Could you check a few things on this model? Use its own coordinates, in mm. Give positions to 0.01 mm unless a question says otherwise; leave off trailing zeros. Loops run counter-clockwise (first coordinate to the right, second up) from the corner with the lowest first, then second, coordinate; pieces in that order, holes last. Notation, with made-up numbers: M -26,58.5 L 29,58.5 A21 ccw 29,70.5 Z; hole C 22.5,48 d6. An arc over 180 degrees is marked long. Use a Markdown table: item, result. Add a question column.
1) Suppose I cut it at D-D on z = -38. List the corners of the cut face in (x, y) for me.
2) Will these pins go through, and if not, where does the flat tip stop? pin 1 Ø3 at (x, z) = (-26, -39.5) entering from +Y; pin 2 Ø2 at (y, z) = (-1.5, 27.5) entering from -X; pin 3 Ø3 at (y, z) = (-2, -8.5) entering from -X; pin 4 Ø6 at (x, z) = (40.58, 46.87) entering from +Y.
3) Suppose I cut it at A-A on x = 0. List the corners of the cut face in (y, z) for me.
4) If I drill on line 1 along Z through (x, y) = (0, -4.3); line 2 along Z through (x, y) = (0, -2.75); line 3 along Z through (x, y) = (-42.5, -3.3), over which ranges is the centre line in solid material (lowest first)? Write a range as [from, to].
5) Suppose I cut it at C-C on y = -0.8. List the corners of the cut face in (x, z) for me, and give its area (3 significant figures).
6) Suppose I cut it at B-B on z = 0. List the corners of the cut face in (x, y) for me.
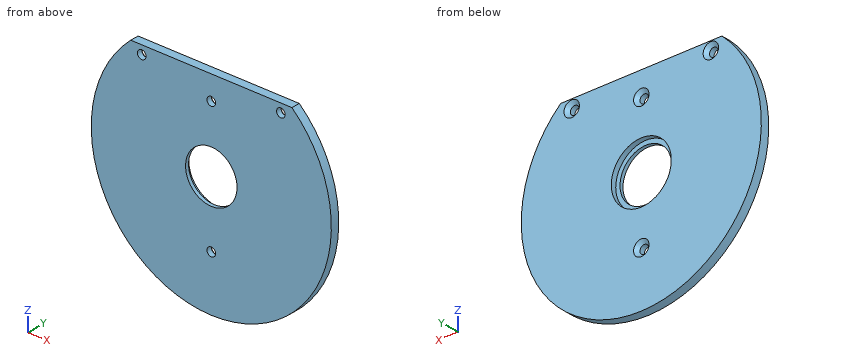
```python
from build123d import *

# Parameters (mm, degrees)
F2_R           = 2.5
F2_R_2         = 17.5
F2_R_3         = 15
F3_DEPTH       = 5
F4_DEPTH       = 3
F5_D           = 5
F5_CSINK_D     = 9
F5_CSINK_ANGLE = 90


with BuildPart() as f3:
    # F2 (on Front) → F3 (new body)
    with BuildSketch(Plane.XZ):
        with BuildLine():
            Line((47, 51.8748493974), (-47, 51.8748493974))
            ThreePointArc((-47, 51.8748493974), (0, -70), (47, 51.8748493974))
        make_face()
        with Locations((0, -38)):
            Circle(F2_R, mode=Mode.SUBTRACT)
        with Locations((-40.5801490137, 46.8748493974)):
            Circle(F2_R, mode=Mode.SUBTRACT)
        Circle(F2_R_2, mode=Mode.SUBTRACT)
        with Locations((0, 38)):
            Circle(F2_R, mode=Mode.SUBTRACT)
        with Locations((40.5801490137, 46.8748493974)):
            Circle(F2_R, mode=Mode.SUBTRACT)
        with Locations((40.5801490137, 46.8748493974)):
            Circle(F2_R)
        with Locations((0, 38)):
            Circle(F2_R)
        with Locations((-40.5801490137, 46.8748493974)):
            Circle(F2_R)
        with Locations((0, -38)):
            Circle(F2_R)
        Circle(F2_R_2)
        Circle(F2_R_3, mode=Mode.SUBTRACT)
    extrude(amount=F3_DEPTH)

    # F2 (on Front) → F4 (cut)
    with BuildSketch(Plane.XZ):
        Circle(F2_R_2)
        Circle(F2_R_3, mode=Mode.SUBTRACT)
    extrude(amount=F4_DEPTH, mode=Mode.SUBTRACT)

    # F5 (through all)
    with Locations(Plane(origin=(0, 0, 0), x_dir=(1, 0, 0), z_dir=(0, 1, 0))):
        with Locations((-40.5801490137, -46.8748493974), (0, -38), (40.5801490137, -46.8748493974), (0, 38)):
            CounterSinkHole(F5_D / 2, F5_CSINK_D / 2, counter_sink_angle=F5_CSINK_ANGLE)


solid = f3.part
```
Answer block:
| question | item | result |
|---|---|---|
| 1 | outline | M -58.79,-5 L -2.5,-5 L -2.5,-2 L -4.5,0 L -58.79,0 Z; M 2.5,-5 L 58.79,-5 L 58.79,0 L 4.5,0 L 2.5,-2 Z |
| 2 | pin 1 | stops at y = 0 |
| 2 | pin 2 | stops at x = -64.79 |
| 2 | pin 3 | stops at x = -69.65 |
| 2 | pin 4 | stops at y = -1.5 |
| 3 | outline | M -5,-70 L 0,-70 L 0,-42.5 L -2,-40.5 L -5,-40.5 Z; M -5,-35.5 L -2,-35.5 L 0,-33.5 L 0,-17.5 L -3,-17.5 L -3,-15 L -5,-15 Z; M -5,15 L -3,15 L -3,17.5 L 0,17.5 L 0,33.5 L -2,35.5 L -5,35.5 Z; M -5,40.5 L -2,40.5 L 0,42.5 L 0,51.87 L -5,51.87 Z |
| 4 | line 1 | z = [-70, -40.5], [-35.5, -15], [15, 35.5], [40.5, 51.87] |
| 4 | line 2 | z = [-70, -40.5], [-35.5, -17.5], [17.5, 35.5], [40.5, 51.87] |
| 4 | line 3 | z = [-55.62, 45.27], [48.48, 51.87] |
| 5 | outline | M -47,51.87 A70 ccw long 47,51.87 Z; hole C -40.58,46.87 d7.4; hole C 0,0 d35; hole C 0,-38 d7.4; hole C 0,38 d7.4; hole C 40.58,46.87 d7.4 |
| 5 | area | 13,100 mm^2 |
| 6 | outline | M -70,-5 L -15,-5 L -15,-3 L -17.5,-3 L -17.5,0 L -70,0 Z; M 15,-5 L 70,-5 L 70,0 L 17.5,0 L 17.5,-3 L 15,-3 Z |
